Work out the finished part from the listing and answer in its coordinate system (mm). Face numbers are marked on the shaded views. A direction names the side the tool comes from. Coordinates: 2 decimals unless noted, no trailing zeros. Order: outer loops, then holes, each group sorted by start corner. A loop starts at its lowest first (then second) coordinate and runs counter-clockwise, first axis right, second up. Notation, with made-up numbers: (12, 55.5) - (18, 55.5) arc R24 cw to (18, 84.5) - close; hole circle Ø10 at (12.5, -4). An arc over 180 degrees is marked (long way). Answer as a JSON object with one key per item and string values. Group by question number.
1) Find the intervals of material crossed by line 1 along X through (y, z) = (-10.5, 22.5); line 2 along Y through (x, z) = (-5.5, 9.5); line 3 along Z through (x, y) = (6.5, -14), in increasing order.
2) Each of these flat-tipped pins is pushed along its axis until it touches: P1, Ø12.5, axis at x = 3.5, y = 16, coming from the +Z side; P2, Ø12, axis at x = -8, y = 2.5, coming from the +Z side. Where does it stop, or does it pass through?
3) A tool of negligible diameter and unlimited length cuts with its end or side. For the marked faces 1 and 2, from which of +Z, -Z, +X, -X, +Y, -Y can it reach the whole face along a straight path? Write none if from no direction.
4) Section C-C (x = -10) is taken. Give the vertices of the cut face in (y, z).
5) The mould has two halves that part along X. Classify the marked faces 3, 4, 5 and 6: released by +X, released by -X, zero draft, split by the parting line, or undercut.
6) Section B-B (y = 20) is taken. Give the vertices of the cut face in (x, z), plus the area to 3 significant figures.
7) Section A-A (z = 10.5) is taken. Give the vertices of the cut face in (x, y).
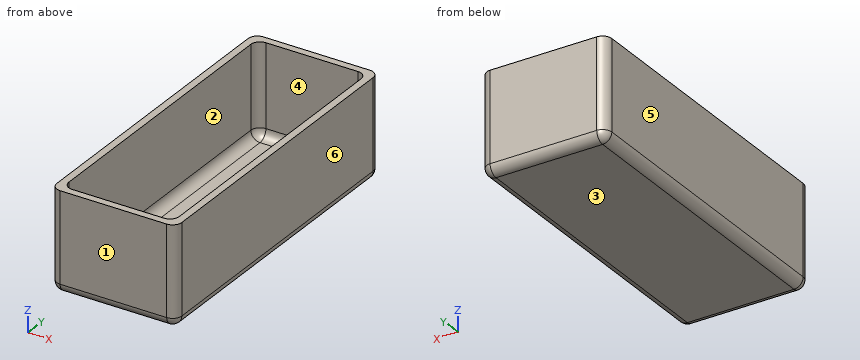
from build123d import *

# Parameters (mm, degrees)
ESQUISSE1_W        = 30
ESQUISSE1_H        = 82
BOSS_EXTRU_1_DEPTH = 25
COQUE1_T           = 2
CONG_1_R           = 2.5


with BuildPart() as part:
    # Esquisse1 → Boss.-Extru.1 (new body)
    with BuildSketch(Plane.XY):
        Rectangle(ESQUISSE1_W, ESQUISSE1_H)
    extrude(amount=BOSS_EXTRU_1_DEPTH)

    # Coque1
    coque1_openings = [part.faces().sort_by_distance(p)[0] for p in [
        (0, 0, 25),
    ]]
    offset(amount=COQUE1_T, openings=coque1_openings, kind=Kind.INTERSECTION)

    # Congé1
    # the kernel refuses this fillet: 2.5 mm, written as the material it adds along each edge
    with BuildSketch(Plane(origin=(-12.5, -38.5, 2.5), x_dir=(-1, 0, 0), z_dir=(0, -1, 0))) as cong_1_piece_1_section:
        Polygon((0, 0), (CONG_1_R, 0), (CONG_1_R, CONG_1_R), (0, CONG_1_R), align=None)
    cong_1_piece_1 = extrude(amount=CONG_1_R, mode=Mode.PRIVATE)
    cong_1_piece_1 = cong_1_piece_1 - Plane(origin=(-12.5, -38.5, 2.5), x_dir=(0.7071067811865475, 0, 0.7071067811865475), z_dir=(0, -1, 0)) * Sphere(CONG_1_R, mode=Mode.PRIVATE)
    add(cong_1_piece_1)
    with BuildSketch(Plane(origin=(-12.5, 38.5, 2.5), x_dir=(0, 1, 0), z_dir=(-1, 0, 0))) as cong_1_piece_2_section:
        Polygon((0, 0), (CONG_1_R, 0), (CONG_1_R, CONG_1_R), (0, CONG_1_R), align=None)
    cong_1_piece_2 = extrude(amount=CONG_1_R, mode=Mode.PRIVATE)
    cong_1_piece_2 = cong_1_piece_2 - Plane(origin=(-12.5, 38.5, 2.5), x_dir=(0, -0.7071067811865475, 0.7071067811865475), z_dir=(-1, 0, 0)) * Sphere(CONG_1_R, mode=Mode.PRIVATE)
    add(cong_1_piece_2)
    with BuildSketch(Plane(origin=(12.5, -38.5, 2.5), x_dir=(1, 0, 0), z_dir=(0, -1, 0))) as cong_1_piece_3_section:
        Polygon((0, 0), (CONG_1_R, 0), (CONG_1_R, -CONG_1_R), (0, -CONG_1_R), align=None)
    cong_1_piece_3 = extrude(amount=CONG_1_R, mode=Mode.PRIVATE)
    cong_1_piece_3 = cong_1_piece_3 - Plane(origin=(12.5, -38.5, 2.5), x_dir=(-0.7071067811865475, 0, 0.7071067811865475), z_dir=(0, -1, 0)) * Sphere(CONG_1_R, mode=Mode.PRIVATE)
    add(cong_1_piece_3)
    with BuildSketch(Plane(origin=(12.5, 38.5, 2.5), x_dir=(1, 0, 0), z_dir=(0, 1, 0))) as cong_1_piece_4_section:
        Polygon((0, 0), (CONG_1_R, 0), (CONG_1_R, CONG_1_R), (0, CONG_1_R), align=None)
    cong_1_piece_4 = extrude(amount=CONG_1_R, mode=Mode.PRIVATE)
    cong_1_piece_4 = cong_1_piece_4 - Plane(origin=(12.5, 38.5, 2.5), x_dir=(-0.7071067811865475, 0, 0.7071067811865475), z_dir=(0, 1, 0)) * Sphere(CONG_1_R, mode=Mode.PRIVATE)
    add(cong_1_piece_4)
    with BuildSketch(Plane(origin=(-15, -38.5, 0), x_dir=(0, 0, 1), z_dir=(0, 1, 0)), Plane(origin=(15, 38.5, 0), x_dir=(0, 0, 1), z_dir=(0, -1, 0))) as cong_1_piece_5:
        with BuildLine():
            CenterArc((CONG_1_R, CONG_1_R), CONG_1_R, 180, 90)
            Line((0, CONG_1_R), (0, 0))
            Line((0, 0), (CONG_1_R, 0))
        make_face()
    extrude(amount=77)
    with BuildSketch(Plane(origin=(-15, 41, 2.5), x_dir=(0, -1, 0), z_dir=(0, 0, 1)), Plane(origin=(-15, -41, 2.5), x_dir=(1, 0, 0), z_dir=(0, 0, 1)), Plane(origin=(15, 41, 2.5), x_dir=(-1, 0, 0), z_dir=(0, 0, 1))) as cong_1_piece_6:
        with BuildLine():
            CenterArc((CONG_1_R, CONG_1_R), CONG_1_R, 180, 90)
            Line((0, CONG_1_R), (0, 0))
            Line((0, 0), (CONG_1_R, 0))
        make_face()
    extrude(amount=22.5)
    with BuildSketch(Plane(origin=(12.5, -41, 0), x_dir=(0, 0, 1), z_dir=(-1, 0, 0)), Plane(origin=(-12.5, 41, 0), x_dir=(0, 0, 1), z_dir=(1, 0, 0))) as cong_1_piece_7:
        with BuildLine():
            CenterArc((CONG_1_R, CONG_1_R), CONG_1_R, 180, 90)
            Line((0, CONG_1_R), (0, 0))
            Line((0, 0), (CONG_1_R, 0))
        make_face()
    extrude(amount=25)
    with BuildSketch(Plane(origin=(15, -41, 2.5), x_dir=(-1, 0, 0), z_dir=(0, 0, 1))) as cong_1_piece_8:
        with BuildLine():
            CenterArc((CONG_1_R, -CONG_1_R), CONG_1_R, 90, 90)
            Line((0, -CONG_1_R), (0, 0))
            Line((0, 0), (CONG_1_R, 0))
        make_face()
    extrude(amount=22.5)
    # the kernel refuses this fillet: 2.5 mm, written as the material it takes off along each edge
    with BuildSketch(Plane(origin=(14.5, 40.5, 0.5), x_dir=(0, 0, -1), z_dir=(0, 1, 0))) as cong_1_2_piece_1_section:
        Polygon((0, 0), (CONG_1_R, 0), (CONG_1_R, -CONG_1_R), (0, -CONG_1_R), align=None)
    cong_1_2_piece_1 = extrude(amount=CONG_1_R, mode=Mode.PRIVATE)
    cong_1_2_piece_1 = cong_1_2_piece_1 - Plane(origin=(14.5, 40.5, 0.5), x_dir=(-0.7071067811865475, 0, 0.7071067811865475), z_dir=(0, 1, 0)) * Sphere(CONG_1_R, mode=Mode.PRIVATE)
    add(cong_1_2_piece_1, mode=Mode.SUBTRACT)
    with BuildSketch(Plane(origin=(-14.5, 40.5, 0.5), x_dir=(0, 0, -1), z_dir=(0, 1, 0))) as cong_1_2_piece_2_section:
        Polygon((0, 0), (CONG_1_R, 0), (CONG_1_R, CONG_1_R), (0, CONG_1_R), align=None)
    cong_1_2_piece_2 = extrude(amount=CONG_1_R, mode=Mode.PRIVATE)
    cong_1_2_piece_2 = cong_1_2_piece_2 - Plane(origin=(-14.5, 40.5, 0.5), x_dir=(0.7071067811865475, 0, 0.7071067811865475), z_dir=(0, 1, 0)) * Sphere(CONG_1_R, mode=Mode.PRIVATE)
    add(cong_1_2_piece_2, mode=Mode.SUBTRACT)
    with BuildSketch(Plane(origin=(14.5, -40.5, 0.5), x_dir=(1, 0, 0), z_dir=(0, -1, 0))) as cong_1_2_piece_3_section:
        Polygon((0, 0), (CONG_1_R, 0), (CONG_1_R, -CONG_1_R), (0, -CONG_1_R), align=None)
    cong_1_2_piece_3 = extrude(amount=CONG_1_R, mode=Mode.PRIVATE)
    cong_1_2_piece_3 = cong_1_2_piece_3 - Plane(origin=(14.5, -40.5, 0.5), x_dir=(-0.7071067811865475, 0, 0.7071067811865475), z_dir=(0, -1, 0)) * Sphere(CONG_1_R, mode=Mode.PRIVATE)
    add(cong_1_2_piece_3, mode=Mode.SUBTRACT)
    with BuildSketch(Plane(origin=(-14.5, -40.5, 0.5), x_dir=(0, -1, 0), z_dir=(0, 0, -1))) as cong_1_2_piece_4_section:
        Polygon((0, 0), (CONG_1_R, 0), (CONG_1_R, CONG_1_R), (0, CONG_1_R), align=None)
    cong_1_2_piece_4 = extrude(amount=CONG_1_R, mode=Mode.PRIVATE)
    cong_1_2_piece_4 = cong_1_2_piece_4 - Plane(origin=(-14.5, -40.5, 0.5), x_dir=(0.7071067811865475, 0.7071067811865476, 0), z_dir=(0, 0, -1)) * Sphere(CONG_1_R, mode=Mode.PRIVATE)
    add(cong_1_2_piece_4, mode=Mode.SUBTRACT)
    with BuildSketch(Plane(origin=(14.5, 43, -2), x_dir=(0, 0, 1), z_dir=(-1, 0, 0)), Plane(origin=(-14.5, -43, -2), x_dir=(0, 0, 1), z_dir=(1, 0, 0))) as cong_1_2_piece_5:
        with BuildLine():
            CenterArc((CONG_1_R, -CONG_1_R), CONG_1_R, 90, 90)
            Line((0, -CONG_1_R), (0, 0))
            Line((0, 0), (CONG_1_R, 0))
        make_face()
    extrude(amount=29, mode=Mode.SUBTRACT)
    with BuildSketch(Plane(origin=(17, -40.5, -2), x_dir=(0, 0, 1), z_dir=(0, 1, 0)), Plane(origin=(-17, 40.5, -2), x_dir=(0, 0, 1), z_dir=(0, -1, 0))) as cong_1_2_piece_6:
        with BuildLine():
            CenterArc((CONG_1_R, -CONG_1_R), CONG_1_R, 90, 90)
            Line((0, -CONG_1_R), (0, 0))
            Line((0, 0), (CONG_1_R, 0))
        make_face()
    extrude(amount=81, mode=Mode.SUBTRACT)
    with BuildSketch(Plane(origin=(-17, 43, 31.25), x_dir=(1, 0, 0), z_dir=(0, 0, -1)), Plane(origin=(17, -43, 0.5), x_dir=(0, 1, 0), z_dir=(0, 0, 1))) as cong_1_2_piece_7:
        with BuildLine():
            CenterArc((CONG_1_R, CONG_1_R), CONG_1_R, 180, 90)
            Line((0, CONG_1_R), (0, 0))
            Line((0, 0), (CONG_1_R, 0))
        make_face()
    extrude(amount=30.75, mode=Mode.SUBTRACT)
    with BuildSketch(Plane(origin=(17, 43, 31.25), x_dir=(-1, 0, 0), z_dir=(0, 0, -1)), Plane(origin=(-17, -43, 31.25), x_dir=(1, 0, 0), z_dir=(0, 0, -1))) as cong_1_2_piece_8:
        with BuildLine():
            CenterArc((CONG_1_R, -CONG_1_R), CONG_1_R, 90, 90)
            Line((0, -CONG_1_R), (0, 0))
            Line((0, 0), (CONG_1_R, 0))
        make_face()
    extrude(amount=30.75, mode=Mode.SUBTRACT)


solid = part.part
Report:
{
 "1": {"line 1": "x = -17 to -15, 15 to 17", "line 2": "y = -43 to -41, 41 to 43", "line 3": "z = -2 to 0"},
 "2": {"P1": "stops at z = 0", "P2": "stops at z = 0.5"},
 "3": {"face 1": "+Z, -Z, +X, -X, -Y", "face 2": "+Z"},
 "4": {"outline": "(-43, 0.5) arc R2.5 ccw to (-40.5, -2) - (40.5, -2) arc R2.5 ccw to (43, 0.5) - (43, 25) - (41, 25) - (41, 2.5) arc R2.5 cw to (38.5, 0) - (-38.5, 0) arc R2.5 cw to (-41, 2.5) - (-41, 25) - (-43, 25) - close"},
 "5": {"face 3": "zero draft", "face 4": "undercut", "face 5": "released by -X", "face 6": "released by +X"},
 "6": {"outline": "(-17, 0.5) arc R2.5 ccw to (-14.5, -2) - (14.5, -2) arc R2.5 ccw to (17, 0.5) - (17, 25) - (15, 25) - (15, 2.5) arc R2.5 cw to (12.5, 0) - (-12.5, 0) arc R2.5 cw to (-15, 2.5) - (-15, 25) - (-17, 25) - close", "area": "168 mm²"},
 "7": {"outline": "(-17, -40.5) arc R2.5 ccw to (-14.5, -43) - (14.5, -43) arc R2.5 ccw to (17, -40.5) - (17, 40.5) arc R2.5 ccw to (14.5, 43) - (-14.5, 43) arc R2.5 ccw to (-17, 40.5) - close; hole (-15, -38.5) arc R2.5 ccw to (-12.5, -41) - (12.5, -41) arc R2.5 ccw to (15, -38.5) - (15, 38.5) arc R2.5 ccw to (12.5, 41) - (-12.5, 41) arc R2.5 ccw to (-15, 38.5) - close"}
}
